Build history of the part. All positions in model axes, mm. Give positions to 0.01 mm unless a question says otherwise; leave off trailing zeros. Loops run counter-clockwise (first coordinate to the right, second up) from the corner with the lowest first, then second, coordinate; pieces in that order, holes last. Notation, with made-up numbers: (42.25, 70) -> (100.25, 70) arc R32 cw to (100.25, 100) -> close; hole circle Ø6 at (31, -26). An arc over 180 degrees is marked (long way). Answer as a JSON object with one key per item and string values. Group by question number.
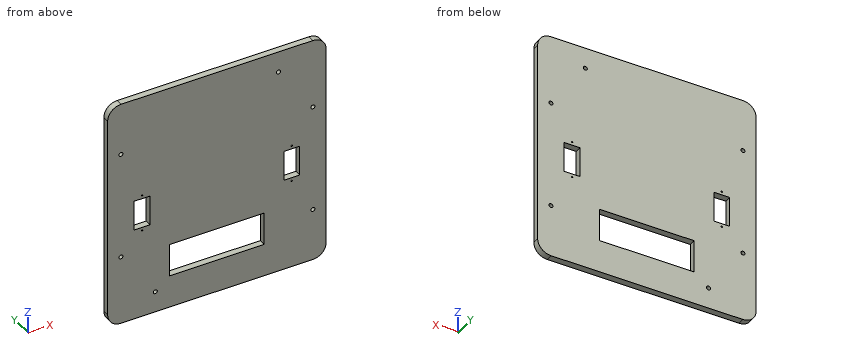
from build123d import *

# Parameters (mm, degrees)
RESSALTO_EXTRUS_O1_DEPTH = 5
ESBO_O2_R                = 1.5
CORTE_EXTRUS_O1_DEPTH    = 5
ESBO_O4_R                = 0.5
ESBO_O4_W                = 12
ESBO_O4_H                = 23
CORTE_EXTRUS_O3_DEPTH    = 193.467750623
ESBO_O5_R                = 1.5
ESBO_O5_W                = 71.5
ESBO_O5_H                = 25
CORTE_EXTRUS_O4_DEPTH    = 193.467750623


with BuildPart() as part:
    # Esboço1 → Ressalto-extrusão1 (new body)
    with BuildSketch(Plane(origin=(0, 0, 0), x_dir=(1, 0, 0), z_dir=(0, 1, 0))):
        with BuildLine():
            Line((-25.463589741, 142.264378701), (119.536410259, 142.264378701))
            ThreePointArc((119.536410259, 142.264378701), (126.607478071, 139.335446513), (129.536410259, 132.264378701))
            Line((129.536410259, 132.264378701), (129.536410259, -22.735621299))
            ThreePointArc((129.536410259, -22.735621299), (126.607478071, -29.806689111), (119.536410259, -32.735621299))
            Line((119.536410259, -32.735621299), (-25.463589741, -32.735621299))
            ThreePointArc((-25.463589741, -32.735621299), (-32.534657553, -29.806689111), (-35.463589741, -22.735621299))
            Line((-35.463589741, -22.735621299), (-35.463589741, 132.264378701))
            ThreePointArc((-35.463589741, 132.264378701), (-32.534657553, 139.335446513), (-25.463589741, 142.264378701))
        make_face()
    extrude(amount=RESSALTO_EXTRUS_O1_DEPTH)

    # Esboço2 → Corte-extrusão1 (cut)
    with BuildSketch(Plane(origin=(0, 5, 0), x_dir=(1, 0, 0), z_dir=(0, 1, 0))):
        with Locations(Location((-25.463589741, 7.264378701, 0), (0, 0, 270))):
            Circle(ESBO_O2_R)
        with Locations(Location((0.536410259, 126.264378701, 0), (0, 0, 270))):
            Circle(ESBO_O2_R)
        with Locations(Location((119.536410259, 102.264378701, 0), (0, 0, 270))):
            Circle(ESBO_O2_R)
        with Locations(Location((93.536410259, -16.735621299, 0), (0, 0, 270))):
            Circle(ESBO_O2_R)
    extrude(amount=-CORTE_EXTRUS_O1_DEPTH, mode=Mode.SUBTRACT)

    # Esboço4 → Corte-extrusão3 (cut, through all)
    with BuildSketch(Plane(origin=(0, 5, 0), x_dir=(1, 0, 0), z_dir=(0, 1, 0))):
        with Locations(Location((-9.463589741, 45.764378701, 0), (0, 0, 270))):
            Circle(ESBO_O4_R)
        with Locations(Location((-9.463589741, 73.764378701, 0), (0, 0, 270))):
            Circle(ESBO_O4_R)
        with Locations(Location((103.536410259, 45.764378701, 0), (0, 0, 270))):
            Circle(ESBO_O4_R)
        with Locations(Location((103.536410259, 73.764378701, 0), (0, 0, 270))):
            Circle(ESBO_O4_R)
        with Locations((-9.463589741, 59.764378701)):
            Rectangle(ESBO_O4_W, ESBO_O4_H)
        with Locations((103.536410259, 59.764378701)):
            Rectangle(ESBO_O4_W, ESBO_O4_H)
    extrude(amount=-CORTE_EXTRUS_O3_DEPTH, mode=Mode.SUBTRACT)

    # Esboço5 → Corte-extrusão4 (cut, through all)
    with BuildSketch(Plane(origin=(0, 5, 0), x_dir=(1, 0, 0), z_dir=(0, 1, 0))):
        with Locations(Location((-25.463589741, 89.264378701, 0), (0, 0, 270))):
            Circle(ESBO_O5_R)
        with Locations(Location((119.536410259, 20.264378701, 0), (0, 0, 270))):
            Circle(ESBO_O5_R)
        with Locations((47.036410259, 104.764378701)):
            Rectangle(ESBO_O5_W, ESBO_O5_H)
    extrude(amount=-CORTE_EXTRUS_O4_DEPTH, mode=Mode.SUBTRACT)


solid = part.part
(1) Saw through at B-B on z = -55.5. List the corners of the cut face in (x, y).
(2) Probe line 1 along X through (y, z) = (4.8, -64); line 2 along Z through (x, y) = (71.5, 1.05); line 3 along X through (y, z) = (0.4, -103). List the from-to ranges inside material, lowest first. Write a range as [from, to].
(3) Saw through at C-C on y = 1.1. Give the number of separate pieces and of enclosed holes in the cut face, plus the area to 3 significant figures.
(4) Pin check, flat tip, straight feed: pin 1 (1.8 mm diameter, centred on x = -25.46, z = -7.26, fed in from +Y). Stop position of the tip, or through.
(5) Saw through at A-A on x = 80. List the corners of the cut face in (y, z), plus the area to 3 significant figures.
Calculated:
{
 "1": {"outline": "(-35.46, 0) -> (-15.46, 0) -> (-15.46, 5) -> (-35.46, 5) -> close; (-3.46, 0) -> (97.54, 0) -> (97.54, 5) -> (-3.46, 5) -> close; (109.54, 0) -> (129.54, 0) -> (129.54, 5) -> (109.54, 5) -> close"},
 "2": {"line 1": "x = [-35.46, -15.46], [-3.46, 97.54], [109.54, 129.54]", "line 2": "z = [-142.26, -117.26], [-92.26, 32.74]", "line 3": "x = [-35.46, 11.29], [82.79, 118.23], [120.84, 129.54]"},
 "3": {"separate pieces": "1", "enclosed holes": "13", "area": "26,400 mm^2"},
 "4": {"pin 1": "passes through"},
 "5": {"outline": "(0, -142.26) -> (5, -142.26) -> (5, -117.26) -> (0, -117.26) -> close; (0, -92.26) -> (5, -92.26) -> (5, 32.74) -> (0, 32.74) -> close", "area": "750 mm^2"}
}
